For this review, take the finished solid that the model builds, in its own axes (mm). Give positions to 0.01 mm unless a question says otherwise; leave off trailing zeros. Loops run counter-clockwise (first coordinate to the right, second up) from the corner with the lowest first, then second, coordinate; pieces in that order, holes last. Notation, with made-up numbers: (19.25, 65) - (64.25, 65) arc R26 ccw to (64.25, 82) - close; hole circle Ø2 at (-30.5, -23). An arc over 180 degrees is marked (long way). Use CSV: the item, a comma, the result in double quotes. Start each with the question number.
1. Mouldability with a two-part tool opening along Y and no side actions: class faces 1 (the flat face through (99, 0, 51)), 2 (the flat face through (99, -1.5, 51)) as pulls with the +Y half, pulls with the -Y half, needs draft (parallel to the pull), parting line crosses it, or undercut.
2. Take a section at A-A on z = 49.5. Give the boundary of the cut face in (x, y), plus the area to 3 significant figures.
3. Take a section at B-B on x = 19. Give the boundary of the cut face in (y, z), plus the area to 4 significant figures.
4. For pin 1 (2.5 mm diameter, centred on x = 15, z = 71, fed in from -Y), flat-tipped, find the tip position at first contact; note if it passes through.
5. Take a section at C-C on y = -1.15. State how many separate pieces and enclosed holes the cut face has, plus the area to 3 significant figures.
6. Wall thickness on line 1 (X direction, y = -1.2, z = 91); line 2 (Z direction, x = 171, y = -0.4); line 3 (Z direction, x = 100, y = -0.55): over which ranges is each line inside the solid? List them lowest first.
```python
from build123d import *

# Parameters (mm, degrees)
F0_W     = 200
F0_H     = 61
F0_W_2   = 40
F0_H_2   = 13
F0_H_3   = 40
F0_R     = 1.5
F1_DEPTH = 1.5


with BuildPart() as f1:
    # F0 (on Front) → F1 (new body)
    with BuildSketch(Plane.XZ):
        with Locations((100, 30.5)):
            Rectangle(F0_W, F0_H)
        with Locations((32.5, 21.5)):
            Rectangle(F0_W_2, F0_H_2, mode=Mode.SUBTRACT)
        with Locations((77.5, 21.5)):
            Rectangle(F0_W_2, F0_H_2, mode=Mode.SUBTRACT)
        with Locations((32.5, 49.5)):
            Rectangle(F0_W_2, F0_H_2, mode=Mode.SUBTRACT)
        with Locations((77.5, 49.5)):
            Rectangle(F0_W_2, F0_H_2, mode=Mode.SUBTRACT)
        with Locations((122.5, 21.5)):
            Rectangle(F0_W_2, F0_H_2, mode=Mode.SUBTRACT)
        with Locations((167.5, 21.5)):
            Rectangle(F0_W_2, F0_H_2, mode=Mode.SUBTRACT)
        with Locations((122.5, 49.5)):
            Rectangle(F0_W_2, F0_H_2, mode=Mode.SUBTRACT)
        with Locations((167.5, 49.5)):
            Rectangle(F0_W_2, F0_H_2, mode=Mode.SUBTRACT)
        with Locations((100, 81)):
            Rectangle(F0_W, F0_H_3)
        with Locations((15, 71)):
            Circle(F0_R, mode=Mode.SUBTRACT)
        with Locations((15, 91)):
            Circle(F0_R, mode=Mode.SUBTRACT)
        with Locations((100, 71)):
            Circle(F0_R, mode=Mode.SUBTRACT)
        with Locations((185, 71)):
            Circle(F0_R, mode=Mode.SUBTRACT)
        with Locations((100, 91)):
            Circle(F0_R, mode=Mode.SUBTRACT)
        with Locations((185, 91)):
            Circle(F0_R, mode=Mode.SUBTRACT)
    extrude(amount=F1_DEPTH)


solid = f1.part
```
Check result:
1,face 1,"pulls with the +Y half"
1,face 2,"pulls with the -Y half"
2,outline,"(0, -1.5) - (12.5, -1.5) - (12.5, 0) - (0, 0) - close; (52.5, -1.5) - (57.5, -1.5) - (57.5, 0) - (52.5, 0) - close; (97.5, -1.5) - (102.5, -1.5) - (102.5, 0) - (97.5, 0) - close; (142.5, -1.5) - (147.5, -1.5) - (147.5, 0) - (142.5, 0) - close; (187.5, -1.5) - (200, -1.5) - (200, 0) - (187.5, 0) - close"
2,area,"60.0 mm²"
3,outline,"(-1.5, 0) - (0, 0) - (0, 15) - (-1.5, 15) - close; (-1.5, 28) - (0, 28) - (0, 43) - (-1.5, 43) - close; (-1.5, 56) - (0, 56) - (0, 101) - (-1.5, 101) - close"
3,area,"112.5 mm²"
4,pin 1,"passes through"
5,separate pieces,"1"
5,enclosed holes,"14"
5,area,"16,000 mm²"
6,line 1,"x = 0 to 13.5, 16.5 to 98.5, 101.5 to 183.5, 186.5 to 200"
6,line 2,"z = 0 to 15, 28 to 43, 56 to 101"
6,line 3,"z = 0 to 69.5, 72.5 to 89.5, 92.5 to 101"
